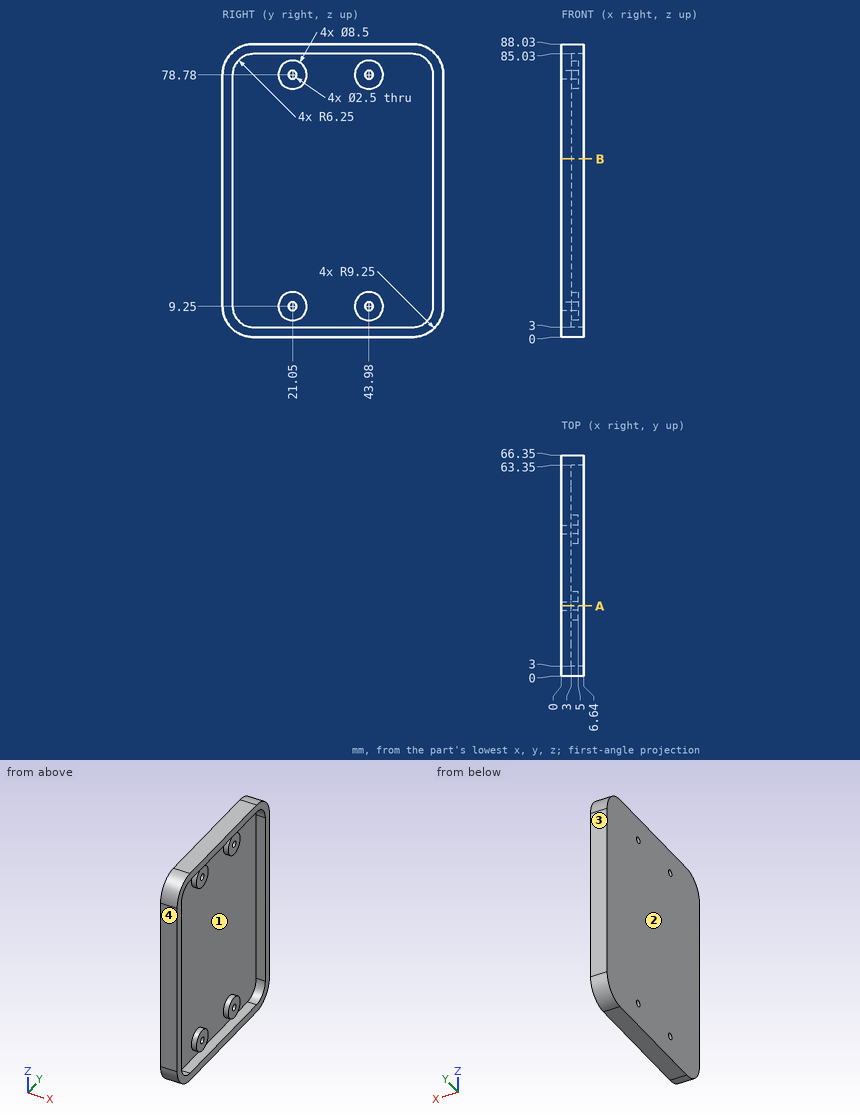
Geometry check sheet. Reference: drawing and pictorial views, mm from the part's lowest x, y, z. Coordinates: 2 decimals unless noted, no trailing zeros. Write each loop counter-clockwise with the first axis right and the second up, starting at its lowest first coordinate (ties: lowest second). Pieces come first, ordered by that corner, then holes. Notation, with made-up numbers: M 6.5,51.5 L 39.5,51.5 A10 cw 39.5,60.5 Z; hole C -15,15.5 d4. An arc over 180 degrees is marked long. Write item = value, one per line. Start each with the question number.
1. Go/stop test with flat-tipped pins: pin 1 (10 mm diameter, centred on y = 9.5, z = 32, fed in from +X); pin 2 (4 mm diameter, centred on y = 45.5, z = 78, fed in from +X); pin 3 (2 mm diameter, centred on y = 21.05, z = 9.25, fed in from +X). Record where each tip stops, or that it passes through.
2. Thickness scan on probe 1 along Y at (x, z) = (0.85, 78.78); probe 2 along Y at (x, z) = (4.4, 78.78); probe 3 along Y at (x, z) = (5.25, 41). Record the ranges inside material, lowest first.
3. Mould release check, pull along Y, two halves, no side actions. Record for the marked faces 1, 2, 3 and 4: pulls with the +Y half, pulls with the -Y half, needs draft (parallel to the pull), parting line crosses it, or undercut.
4. Sectioned sample at A-A (y = 21.05). Record the cut outline in (x, z).
5. Sectioned sample at B-B (z = 53.5). Record the cut outline in (x, y).
The answers:
q1.pin_1 = 3
q1.pin_2 = 5
q1.pin_3 = through
q2.probe_1 = 0 to 19.8, 22.3 to 42.73, 45.23 to 66.35
q2.probe_2 = 0 to 3, 16.8 to 19.8, 22.3 to 25.3, 39.73 to 42.73, 45.23 to 48.23, 63.35 to 66.35
q2.probe_3 = 0 to 3, 63.35 to 66.35
q3.face_1 = undercut
q3.face_2 = needs draft
q3.face_3 = pulls with the +Y half
q3.face_4 = pulls with the -Y half
q4.outline = M 0,0 L 6.64,0 L 6.64,3 L 3,3 L 3,5 L 5,5 L 5,8 L 0,8 Z; M 0,10.5 L 5,10.5 L 5,13.5 L 3,13.5 L 3,74.53 L 5,74.53 L 5,77.53 L 0,77.53 Z; M 0,80.03 L 5,80.03 L 5,83.03 L 3,83.03 L 3,85.03 L 6.64,85.03 L 6.64,88.03 L 0,88.03 Z
q5.outline = M 0,0 L 6.64,0 L 6.64,3 L 3,3 L 3,63.35 L 6.64,63.35 L 6.64,66.35 L 0,66.35 Z
